from build123d import *

# Parameters (mm, degrees)
SKETCH1_W            = 59.902393064
SKETCH1_H            = 59.902393064
SKETCH1_W_2          = 55.902393064
SKETCH1_H_2          = 55.902393064
SKETCH1_W_3          = 5
SKETCH1_H_3          = 5
SKETCH1_H_4          = 5.157397932
SKETCH1_W_4          = 4.976574335
SKETCH1_H_5          = 4.976574335
SKETCH1_W_5          = 4.983582997
SKETCH1_H_6          = 4.983582997
BOSS_EXTRUDE1_DEPTH  = 20
BOSS_EXTRUDE2_DEPTH  = 2
SKETCH3_W            = 23
SKETCH3_H            = 1
CUT_EXTRUDE1_DEPTH   = 2
SKETCH4_W            = 29.96
SKETCH4_H            = 59.9024
BOSS_EXTRUDE28_DEPTH = 2
SKETCH5_R            = 1.5
CUT_EXTRUDE2_DEPTH   = 5


with BuildPart() as part:
    # Sketch1 → Boss-Extrude1 (new body)
    with BuildSketch(Plane(origin=(0, 0, 0), x_dir=(1, 0, 0), z_dir=(0, 1, 0))):
        Rectangle(SKETCH1_W, SKETCH1_H)
        Rectangle(SKETCH1_W_2, SKETCH1_H_2, mode=Mode.SUBTRACT)
        with Locations((-25.451196532, 25.451196532)):
            Rectangle(SKETCH1_W_3, SKETCH1_H_3)
        with Locations((25.451196532, 25.372497566)):
            Rectangle(SKETCH1_W_3, SKETCH1_H_4)
        with Locations((25.462909364, -25.462909364)):
            Rectangle(SKETCH1_W_4, SKETCH1_H_5)
        with Locations((-25.459405034, -25.459405034)):
            Rectangle(SKETCH1_W_5, SKETCH1_H_6)
    extrude(amount=BOSS_EXTRUDE1_DEPTH)

    # Sketch2 → Boss-Extrude2 (add)
    with BuildSketch(Plane(origin=(0, 20, 0), x_dir=(1, 0, 0), z_dir=(0, 1, 0))):
        Polygon((4.951196532, -21.090411798), (4.951196532, -0.090411798), (4.951196532, 20.909588202), (4.951196532, 27.951196532), (0, 27.951196532), (0.003504331, -27.951196532), (4.951196532, -27.951196532), align=None)
        Polygon((29.951196532, -21.090411798), (27.951196532, -21.090411798), (27.951196532, -22.974622197), (22.974622197, -22.974622197), (22.974622197, -27.951196532), (4.951196532, -27.951196532), (0.003504331, -27.951196532), (0, -29.951196532), (29.951196532, -29.951196532), align=None)
        Polygon((27.951196532, -22.974622197), (27.951196532, -21.090411798), (4.951196532, -21.090411798), (4.951196532, -27.951196532), (22.974622197, -27.951196532), (22.974622197, -22.974622197), align=None)
        Polygon((27.951196532, 20.909588202), (27.951196532, -0.090411798), (27.951196532, -21.090411798), (29.951196532, -21.090411798), (29.951196532, 20.909588202), align=None)
        Polygon((27.951196532, 22.7937986), (27.951196532, 20.909588202), (29.951196532, 20.909588202), (29.951196532, 29.951196532), (0, 29.951196532), (0, 27.951196532), (4.951196532, 27.951196532), (22.951196532, 27.951196532), (22.951196532, 22.7937986), align=None)
        Polygon((4.951196532, 20.909588202), (27.951196532, 20.909588202), (27.951196532, 22.7937986), (22.951196532, 22.7937986), (22.951196532, 27.951196532), (4.951196532, 27.951196532), align=None)
    extrude(amount=BOSS_EXTRUDE2_DEPTH)

    # Sketch3 → Cut-Extrude1 (cut)
    with BuildSketch(Plane(origin=(0, 22, 0), x_dir=(1, 0, 0), z_dir=(0, 1, 0))):
        with Locations((16.451196532, -23.590411798)):
            Rectangle(SKETCH3_W, SKETCH3_H)
        with Locations((16.451196532, 23.409588202)):
            Rectangle(SKETCH3_W, SKETCH3_H)
    extrude(amount=-CUT_EXTRUDE1_DEPTH, mode=Mode.SUBTRACT)

    # Sketch4 → Boss-Extrude28 (add)
    with BuildSketch(Plane(origin=(0, 20, 0), x_dir=(1, 0, 0), z_dir=(0, 1, 0))):
        with Locations((-14.971196532, -3.468e-06)):
            Rectangle(SKETCH4_W, SKETCH4_H)
    extrude(amount=BOSS_EXTRUDE28_DEPTH)

    # Sketch5 → Cut-Extrude2 (cut)
    with BuildSketch(Plane.XZ):
        with Locations((-26.459405034, 26.459405034)):
            Circle(SKETCH5_R)
        with Locations((26.462909365, 26.462909365)):
            Circle(SKETCH5_R)
        with Locations((26.451196532, -26.372497566)):
            Circle(SKETCH5_R)
        with Locations((-26.451196532, -26.451196532)):
            Circle(SKETCH5_R)
    extrude(amount=-CUT_EXTRUDE2_DEPTH, mode=Mode.SUBTRACT)


solid = part.part
Read the model definition and answer for the solid it produces. Units are mm, in the model's axes. A direction names the side the tool comes from. Coordinates: 2 decimals unless noted, no trailing zeros. Write each loop counter-clockwise with the first axis right and the second up, starting at its lowest first coordinate (ties: lowest second). Pieces come first, ordered by that corner, then holes. Notation, with made-up numbers: (-38.5, 18) - (-20.5, 18) arc R15 cw to (-20.5, 45) - close; hole circle Ø1 at (-10.75, -23). An arc over 180 degrees is marked (long way). One line per question, with ' | ' between items.
Q1. For faces 4 (the flat face through (25, 10, 22.975)), 5 (the flat face through (17, 21, 21.09)), 6 (the flat face through (16, 21, 23.09)), 7 (the flat face through (-29.951, 11, 0)), determine the directions among +Z, -Z, +X, -X, +Y, -Y from which every point of the face is accessible in a straight line to the end or side of a thin tool.
Result set:
face 4: -Y | face 5: +Y, -Y | face 6: +Y | face 7: +Z, -Z, -X, +Y, -Y
Q2. Find section B-B, the plane z = 5. Write down the section's boundary in (x, y).
Result set:
outline: (-29.95, 0) - (-27.95, 0) - (-27.95, 20) - (4.95, 20) - (4.95, 22) - (-29.95, 22) - close; (27.95, 0) - (29.95, 0) - (29.95, 22) - (27.95, 22) - close
Q3. Find section C-C, the plane y = 9. Write down the section's boundary in (x, z).
Result set:
outline: (-29.95, -29.95) - (29.95, -29.95) - (29.95, 29.95) - (-29.95, 29.95) - close; hole (-27.95, -22.95) - (-22.95, -22.95) - (-22.95, -27.95) - (22.95, -27.95) - (22.95, -22.79) - (27.95, -22.79) - (27.95, 22.97) - (22.97, 22.97) - (22.97, 27.95) - (-22.97, 27.95) - (-22.97, 22.97) - (-27.95, 22.97) - close
Q4. Find section A-A, the plane x = 12. Write down the section's boundary in (y, z), plus the area to 3 significant figures.
Result set:
outline: (0, -29.95) - (22, -29.95) - (22, -23.91) - (20, -23.91) - (20, -27.95) - (0, -27.95) - close; (0, 27.95) - (20, 27.95) - (20, 24.09) - (22, 24.09) - (22, 29.95) - (0, 29.95) - close; (20, -22.91) - (22, -22.91) - (22, -20.91) - (20, -20.91) - close; (20, 21.09) - (22, 21.09) - (22, 23.09) - (20, 23.09) - close | area: 112 mm^2
Q5. Determine the mould class of faces 1 (the flat face through (26, 5, -26)), 2 (the flat face through (29.951, 11, 0)), 3 (the flat face through (0, 11, 29.951)) for opening direction Z: +Z half, -Z half, draft (parallel to the pull), parting line (faces both ways), or undercut.
Result set:
face 1: undercut | face 2: draft | face 3: +Z half
Q6. This flat-tipped pin is pushed along its axis until it touches: P1, Ø4, axis at x = -9, z = -16.5, coming from the -Y side. Where does it stop, or does it pass through?
Result set:
P1: y = 20
Q7. Consider L1, parallel to Z at x = -26.5, y = 1.75; L2, parallel to X at y = 18, z = -7; L3, parallel to Z at x = 27, y = 20.5. Determine where each line is inside the solid, lowest interval first. Write a range as [from, to].
Result set:
L1: [-29.95, -27.95], [-24.95, -22.95], [22.97, 24.96], [27.96, 29.95] | L2: [-29.95, -27.95], [27.95, 29.95] | L3: [-29.95, -23.91], [-22.91, -20.91], [21.09, 23.09], [24.09, 29.95]
